Here's how the part is built. I have some questions about the finished solid (model axes, mm). A direction names the side the tool comes from. Coordinates: 2 decimals unless noted, no trailing zeros. Write each loop counter-clockwise with the first axis right and the second up, starting at its lowest first coordinate (ties: lowest second). Pieces come first, ordered by that corner, then holes.
```python
from build123d import *

# Parameters (mm, degrees)
F2_SIZE  = 1
F4_DEPTH = 20
F5_R     = 2.5
F5_R_2   = 1.5
F6_DEPTH = 17.001


with BuildPart() as f1:
    # F0 (on Front) → F1 (revolve)
    with BuildSketch(Plane.XZ):
        Polygon((-53, 0), (0, 0), (20, 0), (20, 10), (0, 10), (0, 5), (-2, 5), (-2, 4), (-50, 4), (-50, 3), (-50.9, 3), (-50.9, 4), (-53, 4), align=None)
    revolve(axis=Axis((-15.901639617, 0, 0), (1, 0, 0)))

    # F2
    f2_edges = [f1.edges().sort_by_distance(p)[0] for p in [
        (-53, 0, -4),
        (20, 0, -10),
    ]]
    chamfer(f2_edges, length=F2_SIZE)

    # F3 (on face) → F4 (cut, through all)
    with BuildSketch(Plane.YZ.offset(20)):
        with BuildLine():
            Line((-7, -7.1414284285), (-7, 7.1414284285))
            ThreePointArc((-7, 7.1414284285), (-10, 0), (-7, -7.1414284285))
        make_face()
    extrude(amount=-F4_DEPTH, mode=Mode.SUBTRACT)

    # F5 (on face) → F6 (cut, through all)
    with BuildSketch(Plane.XZ.offset(7)):
        with Locations((10, 0)):
            Circle(F5_R)
        with Locations((-25, 0)):
            Circle(F5_R_2)
    extrude(amount=-F6_DEPTH, mode=Mode.SUBTRACT)


solid = f1.part
```
1) We'd pull the mould along X, two halves only. Please class faces 4 (the face through (19.826, 9.168, -0.316)), 5 (the face through (-50.5, -0.1, -3)), 6 (the face through (-51.458, 3.905, -0.867)): pulls with the +X half, pulls with the -X half, needs draft (parallel to the pull), parting line crosses it, or undercut.
Values follow:
face 4: pulls with the +X half
face 5: undercut
face 6: needs draft
2) On a 3-axis mill with a long thin cutter (end or side, diameter ignored), from which of +Z, -Z, +X, -X, +Y, -Y can I reach the whole of each face in a straight line? I mean faces 1 (the face through (-50.9, -3, -1)), 2 (the face through (-26.336, 3.549, 1.846)), 3 (the face through (20, 1, 0)). Say none if no direction works.
Values follow:
face 1: none
face 2: -X
face 3: +Z, -Z, +X, +Y, -Y
3) Imagine slicing it at C-C on x = -25. Please give me the cut outline in (y, z), then the cut area to 3 significant figures.
Values follow:
outline: (-3.71, -1.5) arc R4 ccw to (3.71, -1.5) - close; (-3.71, 1.5) - (3.71, 1.5) arc R4 ccw to start
area: 26.8 mm2
4) Imagine slicing it at A-A on z = 0. Count the separate pieces of the cut face and the enclosed holes in it, then the cut area to 3 significant figures.
Values follow:
separate pieces: 3
enclosed holes: 0
area: 656 mm2
5) I need wall thicknesses on probe 1 along X at (y, z) = (1, 0); probe 2 along X at (y, z) = (3.25, 0.5); probe 3 along X at (y, z) = (1, 1). Which ranges of each line are inside material? Lowest first, please.
Values follow:
probe 1: x = -53 to -26.5, -23.5 to 7.5, 12.5 to 20
probe 2: x = -52.71 to -50.9, -50 to -26.41, -23.59 to 7.55, 12.45 to 20
probe 3: x = -53 to -26.12, -23.88 to 7.71, 12.29 to 20
6) Will these pins go through, and if not, where does the flat tip stop? pin 1 (6 mm diameter, centred on x = 9, y = -4, fed in from +Z); pin 2 (8 mm diameter, centred on x = -33.5, y = 7.5, fed in from -Z); pin 3 (3 mm diameter, centred on x = -27, y = 0.5, fed in from -Z).
Values follow:
pin 1: stops at z = 9.95
pin 2: stops at z = -1.94
pin 3: stops at z = -4
7) Imagine slicing it at B-B on x = 6.5. Please give me the cut outline in (y, z), then the cut area to 3 significant figures.
Values follow:
outline: (-7, -7.14) arc R10 ccw (long way) to (-7, 7.14) - close
area: 285 mm2
